For this review, take the finished solid that the model builds, in its own axes (mm). Face numbers are marked on the shaded views. A direction names the side the tool comes from. Give positions to 0.01 mm unless a question says otherwise; leave off trailing zeros. Loops run counter-clockwise (first coordinate to the right, second up) from the corner with the lowest first, then second, coordinate; pieces in that order, holes last. Notation, with made-up numbers: (-38, 83.5) - (17, 83.5) arc R16 cw to (17, 104.5) - close; hole circle Ø6 at (48, -32). An arc over 180 degrees is marked (long way). Answer as CSV lines item,"result".
from build123d import *

# Parameters (mm, degrees)
SKETCH1_W           = 261.62
SKETCH1_H           = 203.2
BOSS_EXTRUDE1_DEPTH = 5.08
BOSS_EXTRUDE3_DEPTH = 55.88
BOSS_EXTRUDE4_DEPTH = 11.176
SKETCH7_W           = 251.46
SKETCH7_H           = 116.84
BOSS_EXTRUDE5_DEPTH = 11.176
SKETCH8_R           = 5.08
CUT_EXTRUDE2_DEPTH  = 11.176
CUT_EXTRUDE3_DEPTH  = 11.176
SKETCH10_W          = 82.55
SKETCH10_H          = 59.69
CUT_EXTRUDE4_DEPTH  = 5.08
SKETCH12_R          = 1.27
CUT_EXTRUDE5_DEPTH  = 8.89
SKETCH13_W          = 96.52
SKETCH13_H          = 66.04
CUT_EXTRUDE6_DEPTH  = 3.81
SKETCH14_W          = 251.46
SKETCH14_H          = 5.08
BOSS_EXTRUDE6_DEPTH = 44.704
CUT_EXTRUDE7_DEPTH  = 39.624
CUT_EXTRUDE8_DEPTH  = 39.624
CUT_EXTRUDE9_DEPTH  = 39.624
FILLET1_R           = 2.54


with BuildPart() as part:
    # Sketch1 → Boss-Extrude1 (new body)
    with BuildSketch(Plane(origin=(0, 0, 0), x_dir=(1, 0, 0), z_dir=(0, 1, 0))):
        with Locations((130.81, 101.6)):
            Rectangle(SKETCH1_W, SKETCH1_H)
    extrude(amount=BOSS_EXTRUDE1_DEPTH)

    # Sketch4 → Boss-Extrude3 (add)
    with BuildSketch(Plane(origin=(0, 5.08, 0), x_dir=(1, 0, 0), z_dir=(0, 1, 0))):
        Polygon((0, 0), (5.08, 0), (5.08, 198.12), (256.54, 198.12), (256.54, 0), (261.62, 0), (261.62, 203.2), (0, 203.2), align=None)
    extrude(amount=BOSS_EXTRUDE3_DEPTH)

    # Sketch5 → Boss-Extrude4 (add)
    with BuildSketch(Plane(origin=(0, 5.08, 0), x_dir=(1, 0, 0), z_dir=(0, 1, 0))):
        Polygon((5.08, 121.92), (124.46, 121.92), (124.46, 198.12), (137.16, 198.12), (137.16, 121.92), (256.54, 121.92), (256.54, 116.84), (5.08, 116.84), align=None)
    extrude(amount=BOSS_EXTRUDE4_DEPTH)

    # Sketch7 → Boss-Extrude5 (add)
    with BuildSketch(Plane(origin=(0, 5.08, 0), x_dir=(1, 0, 0), z_dir=(0, 1, 0))):
        with Locations((130.81, 58.42)):
            Rectangle(SKETCH7_W, SKETCH7_H)
    extrude(amount=BOSS_EXTRUDE5_DEPTH)

    # Sketch8 → Cut-Extrude2 (cut)
    with BuildSketch(Plane.XY.offset(-198.12)):
        with Locations((17.78, 45.72)):
            Circle(SKETCH8_R)
        with Locations((151.4856, 45.72)):
            Circle(SKETCH8_R)
    extrude(amount=-CUT_EXTRUDE2_DEPTH, mode=Mode.SUBTRACT)

    # Sketch9 → Cut-Extrude3 (cut)
    with BuildSketch(Plane(origin=(5.08, 0, 0), x_dir=(0, 0, -1), z_dir=(1, 0, 0))):
        with BuildLine():
            Line((52.07, 16.256), (64.77, 16.256))
            ThreePointArc((64.77, 16.256), (65.668025612, 16.627974388), (66.04, 17.526))
            Line((66.04, 17.526), (66.04, 23.876))
            ThreePointArc((66.04, 23.876), (65.668025612, 24.774025612), (64.77, 25.146))
            Line((64.77, 25.146), (52.07, 25.146))
            ThreePointArc((52.07, 25.146), (51.171974388, 24.774025612), (50.8, 23.876))
            Line((50.8, 23.876), (50.8, 17.526))
            ThreePointArc((50.8, 17.526), (51.171974388, 16.627974388), (52.07, 16.256))
        make_face()
    extrude(amount=-CUT_EXTRUDE3_DEPTH, mode=Mode.SUBTRACT)

    # Sketch10 → Cut-Extrude4 (cut)
    with BuildSketch(Plane(origin=(0, 16.256, 0), x_dir=(1, 0, 0), z_dir=(0, 1, 0))):
        with Locations((94.615, 46.355)):
            Rectangle(SKETCH10_W, SKETCH10_H)
    extrude(amount=-CUT_EXTRUDE4_DEPTH, mode=Mode.SUBTRACT)

    # Sketch12 → Cut-Extrude5 (cut)
    with BuildSketch(Plane(origin=(0, 11.176, 0), x_dir=(1, 0, 0), z_dir=(0, 1, 0))):
        with Locations(Location((57.15, 72.39, 0), (0, 0, 270))):
            Circle(SKETCH12_R)
        with Locations(Location((57.15, 20.32, 0), (0, 0, 270))):
            Circle(SKETCH12_R)
    extrude(amount=-CUT_EXTRUDE5_DEPTH, mode=Mode.SUBTRACT)

    # Sketch13 → Cut-Extrude6 (cut)
    with BuildSketch(Plane(origin=(0, 16.256, 0), x_dir=(1, 0, 0), z_dir=(0, 1, 0))):
        with Locations((205.74, 76.2)):
            Rectangle(SKETCH13_W, SKETCH13_H)
    extrude(amount=-CUT_EXTRUDE6_DEPTH, mode=Mode.SUBTRACT)

    # Sketch14 → Boss-Extrude6 (add)
    with BuildSketch(Plane(origin=(0, 16.256, 0), x_dir=(1, 0, 0), z_dir=(0, 1, 0))):
        with Locations((130.81, 2.54)):
            Rectangle(SKETCH14_W, SKETCH14_H)
    extrude(amount=BOSS_EXTRUDE6_DEPTH)

    # Sketch15 → Cut-Extrude7 (cut)
    with BuildSketch(Plane(origin=(0, 0, -5.08), x_dir=(-1, 0, 0), z_dir=(0, 0, -1))):
        with BuildLine():
            Line((-106.68, 17.526), (-119.38, 17.526))
            ThreePointArc((-119.38, 17.526), (-120.278025612, 17.897974388), (-120.65, 18.796))
            Line((-120.65, 18.796), (-120.65, 23.876))
            ThreePointArc((-120.65, 23.876), (-120.278025612, 24.774025612), (-119.38, 25.146))
            Line((-119.38, 25.146), (-106.68, 25.146))
            ThreePointArc((-106.68, 25.146), (-105.781974388, 24.774025612), (-105.41, 23.876))
            Line((-105.41, 23.876), (-105.41, 18.796))
            ThreePointArc((-105.41, 18.796), (-105.781974388, 17.897974388), (-106.68, 17.526))
        make_face()
    extrude(amount=-CUT_EXTRUDE7_DEPTH, mode=Mode.SUBTRACT)

    # Sketch16 → Cut-Extrude8 (cut)
    with BuildSketch(Plane.XY):
        with BuildLine():
            Line((161.29, 25.146), (177.8, 25.146))
            ThreePointArc((177.8, 25.146), (178.698025612, 24.774025612), (179.07, 23.876))
            Line((179.07, 23.876), (179.07, 18.796))
            ThreePointArc((179.07, 18.796), (178.698025612, 17.897974388), (177.8, 17.526))
            Line((177.8, 17.526), (161.29, 17.526))
            ThreePointArc((161.29, 17.526), (160.391974388, 17.897974388), (160.02, 18.796))
            Line((160.02, 18.796), (160.02, 23.876))
            ThreePointArc((160.02, 23.876), (160.391974388, 24.774025612), (161.29, 25.146))
        make_face()
        with BuildLine():
            Line((29.21, 25.146), (45.72, 25.146))
            ThreePointArc((45.72, 25.146), (46.618025612, 24.774025612), (46.99, 23.876))
            Line((46.99, 23.876), (46.99, 18.796))
            ThreePointArc((46.99, 18.796), (46.618025612, 17.897974388), (45.72, 17.526))
            Line((45.72, 17.526), (29.21, 17.526))
            ThreePointArc((29.21, 17.526), (28.311974388, 17.897974388), (27.94, 18.796))
            Line((27.94, 18.796), (27.94, 23.876))
            ThreePointArc((27.94, 23.876), (28.311974388, 24.774025612), (29.21, 25.146))
        make_face()
    extrude(amount=-CUT_EXTRUDE8_DEPTH, mode=Mode.SUBTRACT)

    # Sketch17 → Cut-Extrude9 (cut)
    with BuildSketch(Plane.ZY.offset(-256.54)):
        with BuildLine():
            Line((-166.37, 38.1), (-148.59, 38.1))
            ThreePointArc((-148.59, 38.1), (-147.691974388, 37.728025612), (-147.32, 36.83))
            Line((-147.32, 36.83), (-147.32, 20.32))
            ThreePointArc((-147.32, 20.32), (-147.691974388, 19.421974388), (-148.59, 19.05))
            Line((-148.59, 19.05), (-166.37, 19.05))
            ThreePointArc((-166.37, 19.05), (-167.268025612, 19.421974388), (-167.64, 20.32))
            Line((-167.64, 20.32), (-167.64, 36.83))
            ThreePointArc((-167.64, 36.83), (-167.268025612, 37.728025612), (-166.37, 38.1))
        make_face()
    extrude(amount=-CUT_EXTRUDE9_DEPTH, mode=Mode.SUBTRACT)

    # Fillet1
    fillet1_edges = [part.edges().sort_by_distance(p)[0] for p in [
        (0, 30.48, -203.2),
        (261.62, 30.48, -203.2),
        (261.62, 30.48, 0),
        (0, 30.48, 0),
    ]]
    fillet(fillet1_edges, radius=FILLET1_R)


solid = part.part
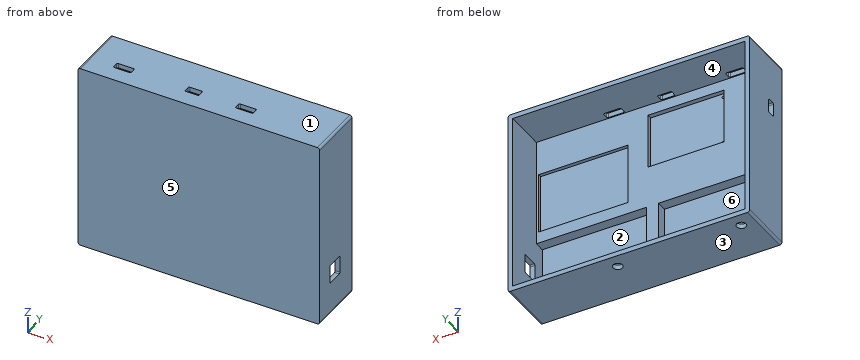
1) Insertion check: P1, Ø9, axis at x = 17.78, y = 45.72, coming from the -Z side; P2, Ø4, axis at x = 196, z = -138.5, coming from the +Y side; P3, Ø4, axis at x = 100.5, z = -110, coming from the +Y side. Each pin has a flat end and moves straight along its axis. Give the tip position at first contact, or say it passes through.
From the geometry:
P1,"stops at z = -5.08"
P2,"stops at y = 5.08"
P3,"stops at y = 16.26"
2) Consider section B-B on y = 45.72. Write out the cut boundary in (x, z), and give its area (3 significant figures).
From the geometry:
outline,"(0, -200.66) arc R2.54 ccw to (2.54, -203.2) - (12.7, -203.2) - (12.7, -198.12) - (5.08, -198.12) - (5.08, -5.08) - (256.54, -5.08) - (256.54, -198.12) - (156.57, -198.12) - (156.57, -203.2) - (259.08, -203.2) arc R2.54 ccw to (261.62, -200.66) - (261.62, -2.54) arc R2.54 ccw to (259.08, 0) - (2.54, 0) arc R2.54 ccw to (0, -2.54) - close; (22.86, -203.2) - (146.41, -203.2) - (146.41, -198.12) - (22.86, -198.12) - close"
area,"4,510 mm^2"
3) Draft analysis for pull direction Z (two halves, no side actions). For the marked faces 3, 4, 5 and 6, state which applies: pulls with the +Z half, pulls with the -Z half, needs draft (parallel to the pull), parting line crosses it, or undercut.
From the geometry:
face 3,"pulls with the -Z half"
face 4,"undercut"
face 5,"needs draft"
face 6,"undercut"
4) Consider section A-A on x = 17.78. Write out the cut boundary in (y, z).
From the geometry:
outline,"(0, -203.2) - (40.64, -203.2) - (40.64, -198.12) - (5.08, -198.12) - (5.08, -121.92) - (16.26, -121.92) - (16.26, -5.08) - (60.96, -5.08) - (60.96, 0) - (0, 0) - close; (50.8, -203.2) - (60.96, -203.2) - (60.96, -198.12) - (50.8, -198.12) - close"
5) Wall thickness on line 1 (Z direction, x = 57, y = 7); line 2 (Z direction, x = 45, y = 33.5); line 3 (X direction, y = 51, z = -143): over which ranges is each line inside the solid? List them lowest first. Write a range as from..to.
From the geometry:
line 1,"z = -203.2..-198.12, -121.92..-73.65, -71.13..-21.58, -19.06..0"
line 2,"z = -203.2..-198.12, -5.08..0"
line 3,"x = 0..5.08, 256.54..261.62"
6) Machinability: for the marked faces 1 and 2, which of the approach directions +Z, -Z, +X, -X, +Y, -Y give a long, thin tool a straight path to every point of the face, cutting with its end or side? Answer none if there is none.
From the geometry:
face 1,"+Z, +X, -X, +Y, -Y"
face 2,"+Y"
7) Consider section C-C on z = -191. Write out the cut boundary in (x, y), and give its area (3 significant figures).
From the geometry:
outline,"(0, 0) - (261.62, 0) - (261.62, 60.96) - (256.54, 60.96) - (256.54, 5.08) - (137.16, 5.08) - (137.16, 16.26) - (124.46, 16.26) - (124.46, 5.08) - (5.08, 5.08) - (5.08, 60.96) - (0, 60.96) - close"
area,"2,040 mm^2"
8) Consider section D-D on x = 192. Write out the cut boundary in (y, z).
From the geometry:
outline,"(0, -203.2) - (60.96, -203.2) - (60.96, -198.12) - (5.08, -198.12) - (5.08, -121.92) - (16.26, -121.92) - (16.26, -109.22) - (12.45, -109.22) - (12.45, -43.18) - (16.26, -43.18) - (16.26, -5.08) - (60.96, -5.08) - (60.96, 0) - (0, 0) - close"
